```python
from build123d import *

# Parameters (mm, degrees)
F0_R      = 20
F1_DEPTH  = 25
F2_R      = 10
F3_DEPTH  = 20
F4_R      = 1.55
F5_DEPTH  = 25.001
F6_R      = 3
F7_DEPTH  = 3
F8_R      = 6.5
F9_DEPTH  = 22
F10_W     = 0.5
F10_H     = 21.0267571211
F10_H_2   = 0.5
F10_W_2   = 21.8651188016
F10_W_3   = 23.3558980227
F10_H_3   = 21.8529557288
F11_DEPTH = 20
F12_W     = 0.5
F12_H     = 6.25
F12_W_2   = 6.25
F12_H_2   = 0.5
F13_DEPTH = 22
F14_W     = 2.5
F14_H     = 2.5
F15_DEPTH = 15
F16_DEPTH = 2.001
F17_R     = 1.15
F18_DEPTH = 27.001


with BuildPart() as f1:
    # F0 (on Top) → F1 (new body)
    with BuildSketch(Plane.XY):
        Circle(F0_R)
    extrude(amount=F1_DEPTH)

    # F2 (on face) → F3 (cut)
    with BuildSketch(Plane.XY.offset(25)):
        Circle(F2_R)
    extrude(amount=-F3_DEPTH, mode=Mode.SUBTRACT)

    # F4 (on face) → F5 (cut, through all)
    with BuildSketch(Plane.XY.offset(25)):
        with Locations((10.6066017178, -10.6066017178)):
            Circle(F4_R)
        with Locations((10.6066017178, 10.6066017178)):
            Circle(F4_R)
        with Locations((-10.6066017178, 10.6066017178)):
            Circle(F4_R)
        with Locations((-10.6066017178, -10.6066017178)):
            Circle(F4_R)
    extrude(amount=-F5_DEPTH, mode=Mode.SUBTRACT)

    # F6 (on face) → F7 (cut)
    with BuildSketch(Plane(origin=(0, 0, 0), x_dir=(1, 0, 0), z_dir=(0, 0, -1))):
        with Locations((-10.6066017178, 10.6066017178)):
            Circle(F6_R)
        with Locations((10.6066017178, 10.6066017178)):
            Circle(F6_R)
        with Locations((10.6066017178, -10.6066017178)):
            Circle(F6_R)
        with Locations((-10.6066017178, -10.6066017178)):
            Circle(F6_R)
    extrude(amount=-F7_DEPTH, mode=Mode.SUBTRACT)

    # F8 (on face) → F9 (join)
    with BuildSketch(Plane.XY.offset(5)):
        Circle(F8_R)
    extrude(amount=F9_DEPTH)

    # F10 (on face) → F11 (cut)
    with BuildSketch(Plane.XY.offset(25)):
        with Locations((0, 10.7633785605)):
            Rectangle(F10_W, F10_H)
        Rectangle(F10_W, F10_H_2)
        with Locations((-11.1825594008, 0)):
            Rectangle(F10_W_2, F10_H_2)
        with Locations((11.9279490113, 0)):
            Rectangle(F10_W_3, F10_H_2)
        with Locations((0, -11.1764778644)):
            Rectangle(F10_W, F10_H_3)
    extrude(amount=-F11_DEPTH, mode=Mode.SUBTRACT)

    # F12 (on face) → F13 (cut)
    with BuildSketch(Plane.XY.offset(27)):
        with Locations((0, 3.375)):
            Rectangle(F12_W, F12_H)
        with Locations((3.375, 0)):
            Rectangle(F12_W_2, F12_H_2)
        Rectangle(F12_W, F12_H_2)
        with Locations((-3.375, 0)):
            Rectangle(F12_W_2, F12_H_2)
        with Locations((0, -3.375)):
            Rectangle(F12_W, F12_H)
    extrude(amount=-F13_DEPTH, mode=Mode.SUBTRACT)

    # F14 (on face) → F15 (cut)
    with BuildSketch(Plane.XY.offset(25)):
        Polygon((7.5, 7.5), (7.5, 5), (5, 5), (5, -5), (7.5, -5), (7.5, -7.5), (29.6562510729, -7.5), (29.6562510729, 7.5), align=None)
        with Locations((6.25, 6.25)):
            Rectangle(F14_W, F14_H)
        Polygon((-5, 5), (5, 5), (5, 7.5), (7.5, 7.5), (7.5, 33.6244015744), (-7.5, 33.6244015744), (-7.5, 7.5), (-5, 7.5), align=None)
        Polygon((-5, -5), (-5, 5), (-7.5, 5), (-7.5, 7.5), (-34.9968748779, 7.5), (-34.9968748779, -7.5), (-7.5, -7.5), (-7.5, -5), align=None)
        with Locations((-6.25, 6.25)):
            Rectangle(F14_W, F14_H)
        Polygon((5, -7.5), (5, -5), (-5, -5), (-5, -7.5), (-7.5, -7.5), (-7.5, -35.9319086373), (7.5, -35.9319086373), (7.5, -7.5), align=None)
        with Locations((6.25, -6.25)):
            Rectangle(F14_W, F14_H)
        with Locations((-6.25, -6.25)):
            Rectangle(F14_W, F14_H)
    extrude(amount=-F15_DEPTH, mode=Mode.SUBTRACT)

    # F14 (on face) → F16 (cut, through all)
    with BuildSketch(Plane.XY.offset(25)):
        Polygon((7.5, 7.5), (7.5, 5), (5, 5), (5, -5), (7.5, -5), (7.5, -7.5), (29.6562510729, -7.5), (29.6562510729, 7.5), align=None)
        with Locations((6.25, 6.25)):
            Rectangle(F14_W, F14_H)
        Polygon((-5, 5), (5, 5), (5, 7.5), (7.5, 7.5), (7.5, 33.6244015744), (-7.5, 33.6244015744), (-7.5, 7.5), (-5, 7.5), align=None)
        Polygon((-5, -5), (-5, 5), (-7.5, 5), (-7.5, 7.5), (-34.9968748779, 7.5), (-34.9968748779, -7.5), (-7.5, -7.5), (-7.5, -5), align=None)
        with Locations((-6.25, 6.25)):
            Rectangle(F14_W, F14_H)
        Polygon((5, -7.5), (5, -5), (-5, -5), (-5, -7.5), (-7.5, -7.5), (-7.5, -35.9319086373), (7.5, -35.9319086373), (7.5, -7.5), align=None)
        with Locations((6.25, -6.25)):
            Rectangle(F14_W, F14_H)
        with Locations((-6.25, -6.25)):
            Rectangle(F14_W, F14_H)
    extrude(amount=F16_DEPTH, mode=Mode.SUBTRACT)

    # F17 (on face) → F18 (cut, through all)
    with BuildSketch(Plane(origin=(0, 0, 0), x_dir=(1, 0, 0), z_dir=(0, 0, -1))):
        Circle(F17_R)
    extrude(amount=-F18_DEPTH, mode=Mode.SUBTRACT)


solid = f1.part
```
Source: CAD feature listing. Evaluate the final solid. Frame: model axes, mm. A direction names the side the tool comes from. Coordinates: 2 decimals unless noted, no trailing zeros. Write each loop counter-clockwise with the first axis right and the second up, starting at its lowest first coordinate (ties: lowest second). Pieces come first, ordered by that corner, then holes. Notation, with made-up numbers: (-31.75, 37.5) -> (-10.75, 37.5) arc R25 cw to (-10.75, 67.5) -> close; hole circle Ø9 at (-25.75, -12.5). An arc over 180 degrees is marked (long way). Return JSON: item names as keys, results as strings. Group by question number.
1) Set-up query: faces 4 (the face through (3, -0.25, 16)), 5 (the face through (-2, 5, 18)), 6 (the face through (-6, -2, 10)). Return all of +Z, -Z, +X, -X, +Y, -Y with unobstructed straight access to the full face (end or side cutting, diameter ignored); none if empty.
2) Section query D-D, the plane x = 3.5. Return loops of the section in (y, z), plus the area to 3 significant figures.
3) Contact query for flat-ended pins moving along their axis: P1, Ø3.5, axis at y = -12.5, z = 16.5, coming from the -X side; P2, Ø8, axis at x = -10.61, y = 10.61, coming from the +Z side; P3, Ø12, axis at x = 3.5, y = 9.5, coming from the +Z side; P4, Ø1, axis at x = 12, y = -3.5, coming from the +Z side. Output: stop coordinate, or through.
4) Ray query, line 1 along X through (y, z) = (-4, 25.5); line 2 along X through (y, z) = (-10, 20). Return the intervals inside material, ascending.
5) Mould query, pull axis X, two halves, no side actions, for faces 1 (the face through (-15, 0.25, 8)), 2 (the face through (6, -10, 10)), 3 (the face through (-5, -2, 18)). Classes: +X half, -X half, draft (parallel to the pull), parting line (faces both ways), or undercut.
6) Section query C-C, the plane y = -2. Return loops of the section in (x, z).
7) Section query A-A, the plane x = 16. Return loops of the section in (y, z).
8) Section query B-B, the plane z = 8.5. State how many separate pieces and enclosed holes the cut face has, plus the area to 3 significant figures.
From the geometry:
{
 "1": {"face 4": "+Z, +X, -X", "face 5": "+Z, +X, -X, +Y", "face 6": "+Z, -X, +Y, -Y"},
 "2": {"outline": "(-19.69, 0) -> (19.69, 0) -> (19.69, 10) -> (9.37, 10) -> (9.37, 5) -> (5.48, 5) -> (5.48, 10) -> (5, 10) -> (5, 27) -> (0.25, 27) -> (0.25, 5) -> (-0.25, 5) -> (-0.25, 27) -> (-5, 27) -> (-5, 10) -> (-5.48, 10) -> (-5.48, 5) -> (-9.37, 5) -> (-9.37, 10) -> (-19.69, 10) -> close", "area": "514 mm²"},
 "3": {"P1": "x = -16.87", "P2": "z = 25", "P3": "z = 27", "P4": "z = 10"},
 "4": {"line 1": "-5 to -0.25, 0.25 to 5", "line 2": "-17.32 to -12.03, -9.18 to -7.5, 7.5 to 9.18, 12.03 to 17.32"},
 "5": {"face 1": "draft", "face 2": "undercut", "face 3": "-X half"},
 "6": {"outline": "(-19.9, 0) -> (19.9, 0) -> (19.9, 10) -> (9.8, 10) -> (9.8, 5) -> (6.18, 5) -> (6.18, 10) -> (5, 10) -> (5, 27) -> (0.25, 27) -> (0.25, 5) -> (-0.25, 5) -> (-0.25, 27) -> (-5, 27) -> (-5, 10) -> (-6.18, 10) -> (-6.18, 5) -> (-9.8, 5) -> (-9.8, 10) -> (-19.9, 10) -> close"},
 "7": {"outline": "(-12, 0) -> (12, 0) -> (12, 25) -> (7.5, 25) -> (7.5, 10) -> (0.25, 10) -> (0.25, 5) -> (-0.25, 5) -> (-0.25, 10) -> (-7.5, 10) -> (-7.5, 25) -> (-12, 25) -> close"},
 "8": {"separate pieces": "8", "enclosed holes": "4", "area": "1,010 mm²"}
}
